Input: dimensioned drawing with shaded views. Units: mm. Origin: part minimum x, y, z. A direction names the side the tool comes from. Give positions to 0.01 mm unless a question says otherwise; leave off trailing zeros. Loops run counter-clockwise (first coordinate to the right, second up) from the corner with the lowest first, then second, coordinate; pieces in that order, holes last.
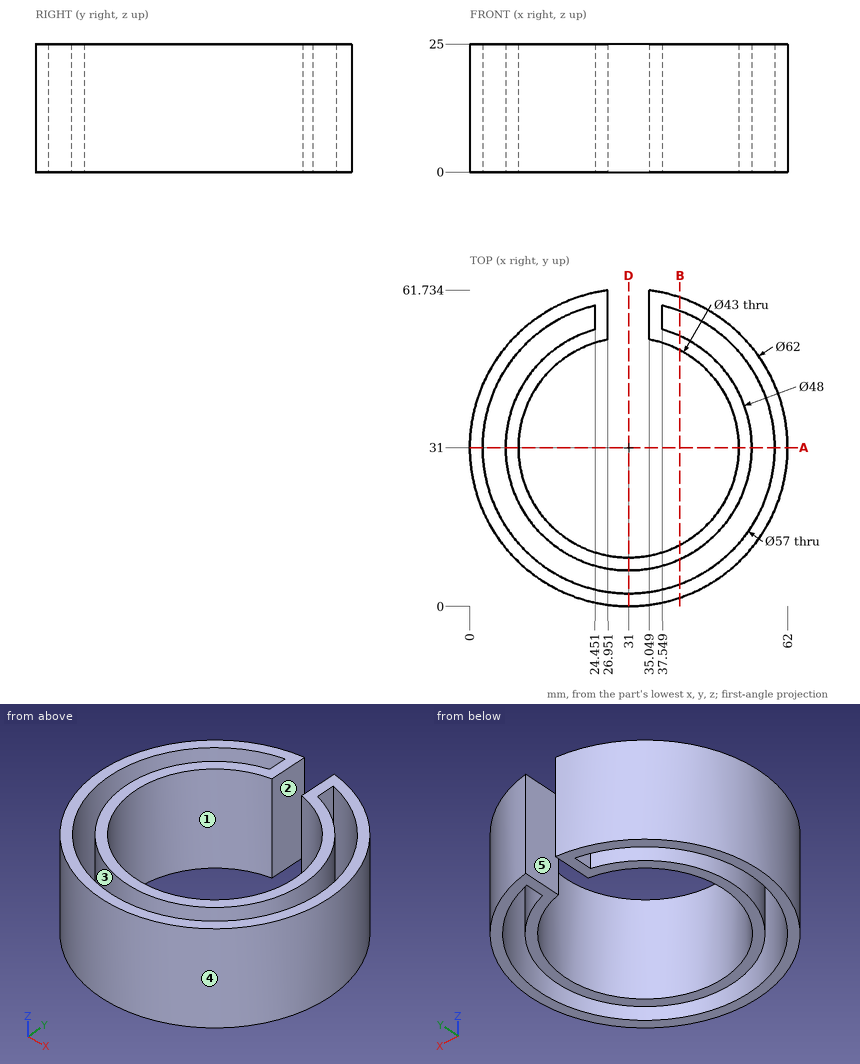
(1) Section D-D, the plane x = 31. Return the cut outline in (y, z).
A:
outline: (0, 0) - (2.5, 0) - (2.5, 25) - (0, 25) - close; (7, 0) - (9.5, 0) - (9.5, 25) - (7, 25) - close
(2) Mould query, pull axis Y, two halves, no side actions, for the marked faces 3, 4 and 5. Classes: pulls with the +Y half, pulls with the -Y half, needs draft (parallel to the pull), parting line crosses it, or undercut.
A:
face 3: undercut
face 4: parting line crosses it
face 5: needs draft
(3) Section B-B, the plane x = 41. Return the cut outline in (y, z), then the cut area to 3 significant figures.
A:
outline: (1.66, 0) - (4.31, 0) - (4.31, 25) - (1.66, 25) - close; (9.18, 0) - (11.97, 0) - (11.97, 25) - (9.18, 25) - close; (50.03, 0) - (52.82, 0) - (52.82, 25) - (50.03, 25) - close; (57.69, 0) - (60.34, 0) - (60.34, 25) - (57.69, 25) - close
area: 272 mm2
(4) First-contact query: pin 1 (1.5 mm diameter, centred on x = 54.5, y = 45.5, fed in from -Z); pin 2 (3 mm diameter, centred on y = 58.5, z = 10.5, fed in from -X); pin 3 (6 mm diameter, centred on y = 10, z = 7, fed in from +X); pin 4 (1 mm diameter, centred on y = 44.5, z = 19, fed in from -X). Flat tips, straight axial feed; report the tip coordinate or a pass-through.
A:
pin 1: passes through
pin 2: stops at x = 14.12
pin 3: stops at x = 56.24
pin 4: stops at x = 2.86
(5) Ray query, line 1 along X through (y, z) = (31, 8); line 2 along Y through (x, z) = (12, 16) (1 decimal); line 3 along Y through (x, z) = (31, 17.5). Return the intervals inside material, ascending.
A:
line 1: x = 0 to 2.5, 7 to 9.5, 52.5 to 55, 59.5 to 62
line 2: y = 6.5 to 9.8, 16.3 to 20.9, 41.1 to 45.7, 52.2 to 55.5
line 3: y = 0 to 2.5, 7 to 9.5
(6) Section A-A, the plane y = 31. Return the cut outline in (x, z).
A:
outline: (0, 0) - (2.5, 0) - (2.5, 25) - (0, 25) - close; (7, 0) - (9.5, 0) - (9.5, 25) - (7, 25) - close; (52.5, 0) - (55, 0) - (55, 25) - (52.5, 25) - close; (59.5, 0) - (62, 0) - (62, 25) - (59.5, 25) - close
(7) Reachability of the marked faces 1 and 2 from +Z, -Z, +X, -X, +Y, -Y: full face, straight path, thin tool, end or side. Return the list, or none.
A:
face 1: +Z, -Z
face 2: +Z, -Z, +Y
